The model under review builds one solid part; all positions refer to its coordinate system, in mm. Face numbers are marked on the shaded views. A direction names the side the tool comes from. Coordinates: 2 decimals unless noted, no trailing zeros. Order: outer loops, then holes, each group sorted by start corner. A loop starts at its lowest first (then second) coordinate and runs counter-clockwise, first axis right, second up. Notation, with made-up numbers: M 54,-12.5 L 91,-12.5 A24 cw 91,8.5 Z; hole C 4.25,35 d1. An arc over 180 degrees is marked long. Answer in a Markdown table with one row per item.
from build123d import *

# Parameters (mm, degrees)
F0_W      = 69.85
F0_H      = 31.75
F1_DEPTH  = 25.4
F2_W      = 44.45
F2_H      = 19.05
F3_DEPTH  = 25.4
F5_DEPTH  = 25.4
F6_R      = 6.6122667184
F7_DEPTH  = 25.4
F9_DEPTH  = 25.4
F11_DEPTH = 25.4


with BuildPart() as f1:
    # F0 (on Front) → F1 (new body)
    with BuildSketch(Plane.XZ):
        with Locations((34.925, 15.875)):
            Rectangle(F0_W, F0_H)
    extrude(amount=F1_DEPTH)

    # F2 (on face) → F3 (cut)
    with BuildSketch(Plane.XZ.offset(25.4)):
        with Locations((47.625, 22.225)):
            Rectangle(F2_W, F2_H)
    extrude(amount=-F3_DEPTH, mode=Mode.SUBTRACT)

    # F4 (on face) → F5 (cut)
    with BuildSketch(Plane.XZ.offset(25.4)):
        with BuildLine():
            ThreePointArc((0, 21.06358689), (12.7, 31.4315601634), (25.4, 21.06358689))
            Line((25.4, 21.06358689), (25.4, 31.75))
            Line((25.4, 31.75), (0, 31.75))
            Line((0, 31.75), (0, 21.06358689))
        make_face()
    extrude(amount=-F5_DEPTH, mode=Mode.SUBTRACT)

    # F6 (on face) → F7 (cut)
    with BuildSketch(Plane.XZ.offset(25.4)):
        with Locations((12.7, 18.469293445)):
            Circle(F6_R)
    extrude(amount=-F7_DEPTH, mode=Mode.SUBTRACT)

    # F8 (on face) → F9 (cut)
    with BuildSketch(Plane.XY.offset(12.7)):
        with BuildLine():
            Line((57.4697845539, -6.35), (32.0697845539, -6.35))
            ThreePointArc((32.0697845539, -6.35), (25.7197845539, -12.7), (32.0697845539, -19.05))
            Line((32.0697845539, -19.05), (57.1458699361, -19.05))
            ThreePointArc((57.1458699361, -19.05), (63.4979349681, -12.8578792423), (57.4697845539, -6.35))
        make_face()
    extrude(amount=-F9_DEPTH, mode=Mode.SUBTRACT)

    # F10 (on face) → F11 (cut)
    with BuildSketch(Plane.XY.offset(12.7)):
        with BuildLine():
            ThreePointArc((59.4271533191, 0), (69.7393281639, -11.6319730082), (62.5223219395, -25.4))
            Line((62.5223219395, -25.4), (69.85, -25.4))
            Line((69.85, -25.4), (69.85, 0))
            Line((69.85, 0), (59.4271533191, 0))
        make_face()
    extrude(amount=F11_DEPTH, mode=Mode.SUBTRACT)


solid = f1.part
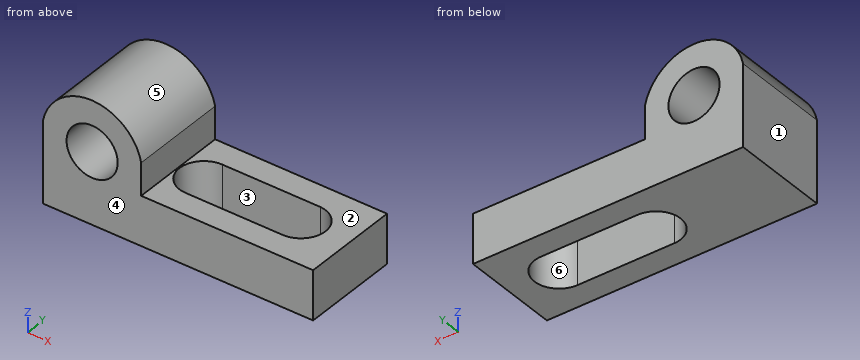
(1) To check wall thickness, follow line 1 (Z direction, x = 12.7, y = -12.25); line 2 (Y direction, x = 51, z = 10); line 3 (Z direction, x = 55.5, y = -20). State the ranges of each line that lie inside material, in increasing order. Write a range as [from, to].
Report:
| item | result |
|---|---|
| line 1 | [0, 11.86], [25.08, 31.43] |
| line 2 | [-25.4, -19.05], [-6.35, 0] |
| line 3 | [0, 12.7] |
(2) Take a section at A-A (x = 40.5). Write out the cut boundary in (y, z), then the cut area to 3 significant figures.
Report:
| item | result |
|---|---|
| outline | M -25.4,0 L -19.05,0 L -19.05,12.7 L -25.4,12.7 Z; M -6.35,0 L 0,0 L 0,12.7 L -6.35,12.7 Z |
| area | 161 mm^2 |
(3) The part is to be moulded in two halves that separate along Y. For the marked faces 4, 5 and 6, say which applies: +Y half, -Y half, draft (parallel to the pull), parting line (faces both ways), or undercut.
Report:
| item | result |
|---|---|
| face 4 | -Y half |
| face 5 | draft |
| face 6 | undercut |
(4) Take a section at B-B (y = -9). Write out the cut boundary in (x, z).
Report:
| item | result |
|---|---|
| outline | M 0,0 L 26.91,0 L 26.91,12.7 L 25.4,12.7 L 25.4,21.06 A12.96 ccw 0,21.06 Z; M 62.31,0 L 69.85,0 L 69.85,12.7 L 62.31,12.7 Z; hole C 12.7,18.47 d13.22 |
(5) Insertion check: P1, Ø4, axis at y = -6.5, z = 16, coming from the +X side; P2, Ø8, axis at y = -3.5, z = 25.5, coming from the +X side; P3, Ø1.5, axis at x = 13, y = -13, coming from the -Z side; P4, Ø12.5, axis at x = 45.5, y = -6.5, coming from the +Z side. Each pin has a flat end and moves straight along its axis. Give the tip position at first contact, or say it passes through.
Report:
| item | result |
|---|---|
| P1 | x = 25.4 |
| P2 | x = 25.3 |
| P3 | z = 0 |
| P4 | z = 12.7 |
(6) Machinability: for the marked faces 1, 2 and 3, which of the approach directions +Z, -Z, +X, -X, +Y, -Y give a long, thin tool a straight path to every point of the face, cutting with its end or side? Answer none if there is none.
Report:
| item | result |
|---|---|
| face 1 | +Z, -Z, -X, +Y, -Y |
| face 2 | +Z, +X, +Y, -Y |
| face 3 | +Z, -Z |
(7) Take a section at C-C (y = -21.5). Write out the cut boundary in (x, z).
Report:
| item | result |
|---|---|
| outline | M 0,0 L 69.85,0 L 69.85,12.7 L 25.4,12.7 L 25.4,21.06 A12.96 ccw 0,21.06 Z; hole C 12.7,18.47 d13.22 |
(8) Take a section at D-D (x = 12.7). Write out the cut boundary in (y, z), then the cut area to 3 significant figures.
Report:
| item | result |
|---|---|
| outline | M -25.4,0 L 0,0 L 0,11.86 L -25.4,11.86 Z; M -25.4,25.08 L 0,25.08 L 0,31.43 L -25.4,31.43 Z |
| area | 462 mm^2 |
